Source: three-view drawing plus pictorial views. Frame: mm from the lowest corner of the part. Coordinates: 2 decimals unless noted, no trailing zeros. Order: outer loops, then holes, each group sorted by start corner. A loop starts at its lowest first (then second) coordinate and runs counter-clockwise, first axis right, second up. Notation, with made-up numbers: (30.25, -11.5) -> (40.25, -11.5) arc R11 ccw to (40.25, 9.5) -> close; hole circle Ø8 at (88.5, 45). An arc over 180 degrees is marked (long way). One line per question, with ' | ' between items.
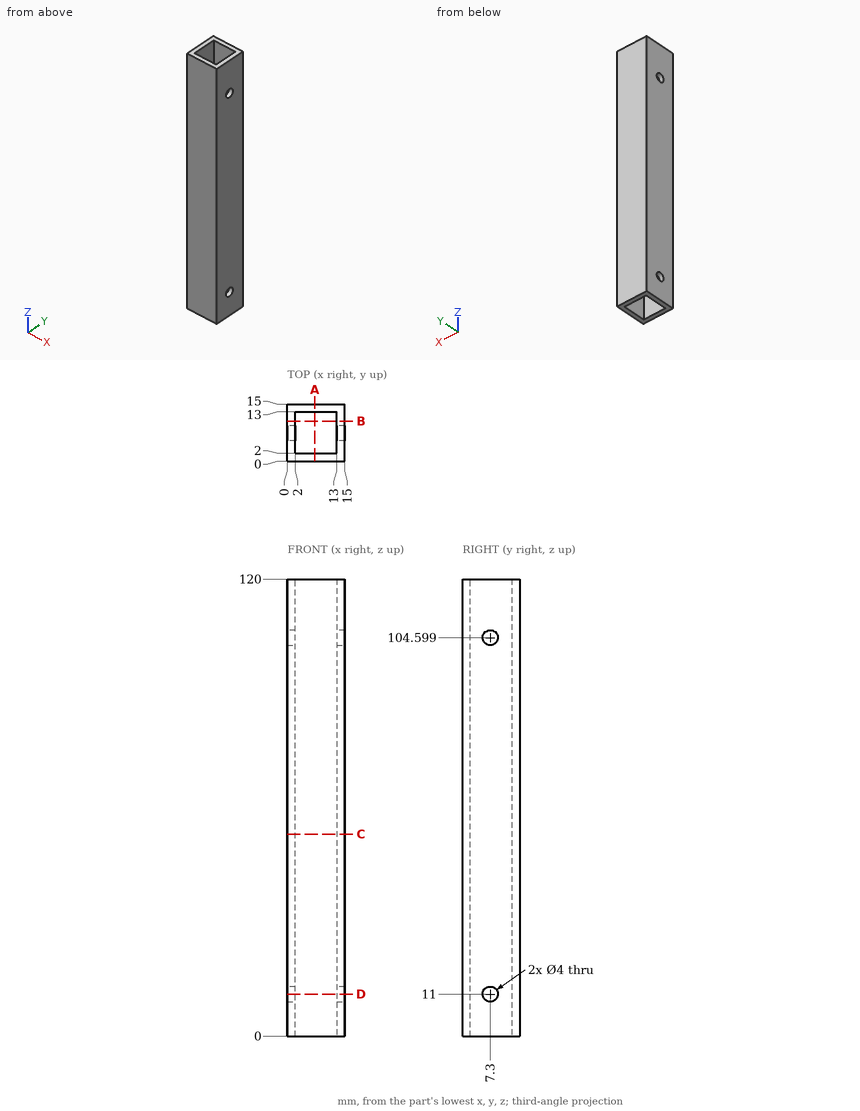
1. Cut plane A-A, the plane x = 7.25. Return loops of the section in (y, z).
Recorded:
outline: (0, 0) -> (2, 0) -> (2, 120) -> (0, 120) -> close; (13, 0) -> (15, 0) -> (15, 120) -> (13, 120) -> close
2. Pin query (flat end, axial travel): pin 1 Ø3.5 at (y, z) = (7.3, 11) entering from +X. Return the tip coordinate at first contact, or that it passes through.
Recorded:
pin 1: passes through
3. Cut plane D-D, the plane z = 11. Return loops of the section in (x, y).
Recorded:
outline: (0, 0) -> (15, 0) -> (15, 5.3) -> (13, 5.3) -> (13, 2) -> (2, 2) -> (2, 5.3) -> (0, 5.3) -> close; (0, 9.3) -> (2, 9.3) -> (2, 13) -> (13, 13) -> (13, 9.3) -> (15, 9.3) -> (15, 15) -> (0, 15) -> close
4. Ray query, line 1 (Z direction, x = 14.05, y = 7.3); line 2 (Y direction, x = 5.5, z = 72.5). Return the intervals inside material, ascending. Write a range as [from, to].
Recorded:
line 1: z = [0, 9], [13, 102.6], [106.6, 120] | line 2: y = [0, 2], [13, 15]
5. Cut plane C-C, the plane z = 53. Return loops of the section in (x, y), and give its area (3 significant figures).
Recorded:
outline: (0, 0) -> (15, 0) -> (15, 15) -> (0, 15) -> close; hole (2, 2) -> (13, 2) -> (13, 13) -> (2, 13) -> close | area: 104 mm^2
